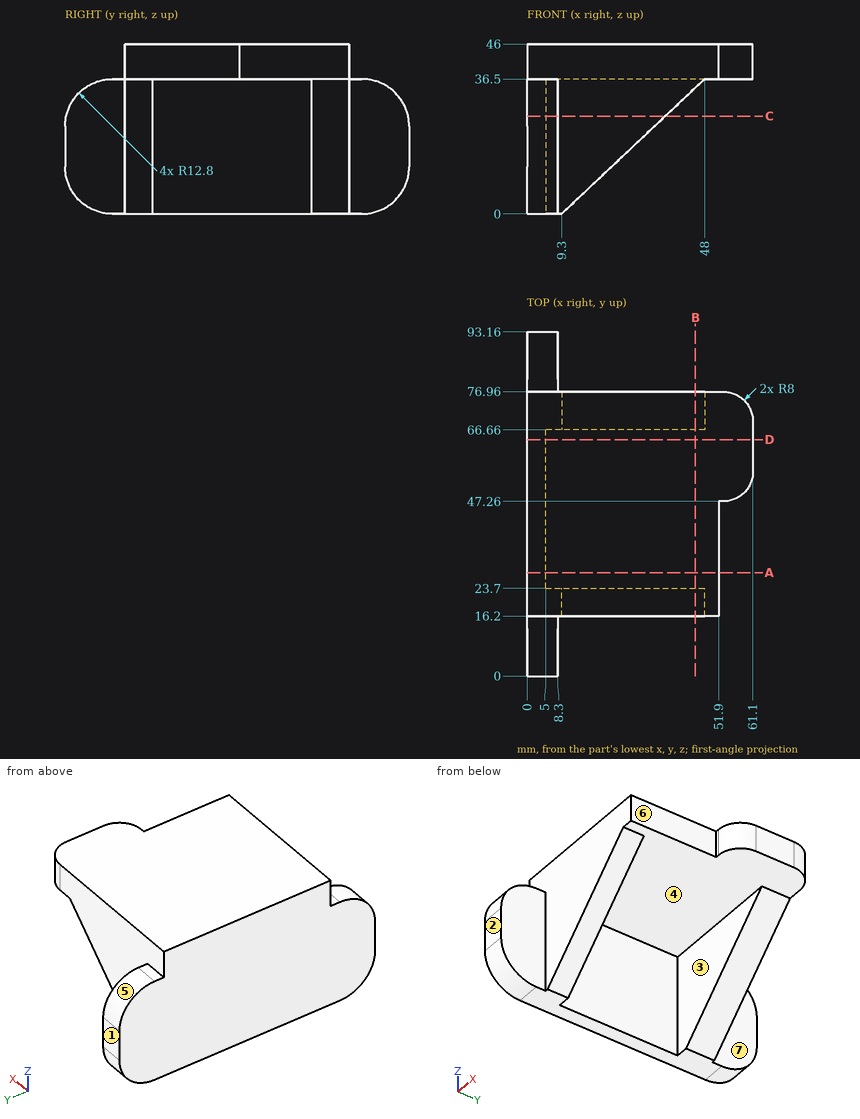
For this review, use the dimensioned drawing (mm, ordinates from the lowest corner) and the shaded views. A direction names the side the tool comes from. Give positions to 0.01 mm unless a question says otherwise; leave off trailing zeros. Order: outer loops, then holes, each group sorted by start corner. A loop starts at its lowest first (then second) coordinate and runs counter-clockwise, first axis right, second up. Notation, with made-up numbers: (2.25, 76.25) - (44.25, 76.25) arc R34 cw to (44.25, 114.25) - close; hole circle Ø9 at (-28.75, -15). An arc over 180 degrees is marked (long way). Use a Markdown table: item, result. Add a question column.
(1) Add section A-A on y = 28. Give the boundary of the cut face in (x, z).
(2) Clearance check with flat-ended pins moving along their axes: P1, Ø6, axis at x = 49, y = 13.5, coming from the -Z side; P2, Ø7.5, axis at y = 28, z = 40, coming from the +X side; P3, Ø12, axis at x = 6, z = 34.5, coming from the +Y side. State where each tip first meets the part, or that it passes through.
(3) Add section D-D on y = 64. Give the boundary of the cut face in (x, z).
(4) Machinability: for the marked faces 4, 5, 6 and 7, which of the approach directions +Z, -Z, +X, -X, +Y, -Y give a long, thin tool a straight path to every point of the face, cutting with its end or side? Answer none if there is none.
(5) Add section C-C on z = 26.5. Give the boundary of the cut face in (x, y), then the cut area to 3 significant figures.
(6) Wall thickness on probe 1 along Y at (x, z) = (20, 20); probe 2 along Y at (x, z) = (46, 44.5); probe 3 along Z at (x, y) = (47.5, 57.5): over which ranges is each line inside the solid? List them lowest first. Write a range as [from, to].
(7) Mouldability with a two-part tool opening along Y and no side actions: class the marked faces 1, 2 and 3 as +Y half, -Y half, draft (parallel to the pull), parting line (faces both ways), or undercut.
(8) Add section B-B on x = 45.5. Give the boundary of the cut face in (y, z).
Report:
| question | item | result |
|---|---|---|
| 1 | outline | (0, 0) - (5, 0) - (5, 36.5) - (51.9, 36.5) - (51.9, 46) - (0, 46) - close |
| 2 | P1 | stops at z = 36.21 |
| 2 | P2 | stops at x = 51.9 |
| 2 | P3 | stops at y = 92.23 |
| 3 | outline | (0, 0) - (5, 0) - (5, 36.5) - (61.1, 36.5) - (61.1, 46) - (0, 46) - close |
| 4 | face 4 | -Z, +X |
| 4 | face 5 | +Z, +X, -X, +Y |
| 4 | face 6 | +Z, -Z, +X, -Y |
| 4 | face 7 | +Z, -Z, +X, +Y |
| 5 | outline | (0, 0.31) - (8.3, 0.31) - (8.3, 16.2) - (37.4, 16.2) - (37.4, 23.7) - (5, 23.7) - (5, 66.66) - (37.4, 66.66) - (37.4, 76.96) - (8.3, 76.96) - (8.3, 92.85) - (0, 92.85) - close |
| 5 | area | 1,140 mm² |
| 6 | probe 1 | y = [16.2, 23.7], [66.66, 76.96] |
| 6 | probe 2 | y = [16.2, 76.96] |
| 6 | probe 3 | z = [36.5, 46] |
| 7 | face 1 | +Y half |
| 7 | face 2 | -Y half |
| 7 | face 3 | undercut |
| 8 | outline | (16.2, 34.14) - (23.7, 34.14) - (23.7, 36.5) - (66.66, 36.5) - (66.66, 34.14) - (76.96, 34.14) - (76.96, 46) - (16.2, 46) - close |
